Model file for the job. Use its own axes, mm. A direction names the side the tool comes from. Round coordinates to 2 decimals unless told otherwise and drop trailing zeros. Order: outer loops, then holes, each group sorted by start corner. A loop starts at its lowest first (then second) coordinate and runs counter-clockwise, first axis right, second up. Notation, with made-up numbers: (57, 10.25) - (69, 10.25) arc R19 ccw to (69, 23.25) - close; hole circle Ø10 at (47.25, 29). An arc over 180 degrees is marked (long way). Answer as CSV lines item,"result". Start each with the question number.
1. 3-axis set-ups, long thin cutter, end or side, ignore diameter. For faces 1 (the face through (-16.026, -11.579, 11.352)), 2 (the face through (-12.5, 0, 27)), 3 (the face through (12.5, 0, 27)): which of +Z, -Z, +X, -X, +Y, -Y reach the whole face in a straight line?
2. Pull direction Y, two halves, no side cores. Call faces 4 (the face through (0, 6.3, 27)), 5 (the face through (18.974, -11.579, 11.352)), 6 (the face through (-8.73, -11.89, 27.48)): released by +Y, released by -Y, zero draft, split by the parting line, or undercut.
3. Band-saw the part on C-C on y = -8.75. List the corners of the cut face in (x, z).
4. Band-saw the part on D-D on y = -5.2. List the corners of the cut face in (x, z).
5. Wall check: line 1 along Z through (x, y) = (-17.5, -10.5); line 2 along X through (y, z) = (-8.75, 37); line 3 along Y through (x, z) = (0, 30). Give the ranges that are in metal, low to high. Write a range as [from, to].
6. Band-saw the part on A-A on z = 10. List the corners of the cut face in (x, y).
7. Pin check, flat tips, straight feed: pin 1 Ø2 at (y, z) = (-3.5, 46) entering from +X; pin 2 Ø2.5 at (x, z) = (-17.5, 10) entering from +Y (3 decimals); pin 3 Ø6.5 at (y, z) = (-2.5, 19.5) entering from -X; pin 4 Ø3 at (x, z) = (15, 29.5) entering from +Y. Stop position of each tip, or through.
```python
from build123d import *

# Parameters (mm, degrees)
SKETCH1_W           = 25
SKETCH1_H           = 23
SKETCH1_R           = 11
SKETCH1_W_2         = 10
SKETCH1_H_2         = 10.1
BOSS_EXTRUDE1_DEPTH = 55.75
SKETCH2_R           = 2
CUT_EXTRUDE1_DEPTH  = 62.487580047


with BuildPart() as part:
    # Sketch1 → Boss-Extrude1 (new body)
    # profile 1 of 3: a face of its own
    with BuildSketch(Plane.XY):
        with Locations((0, -5.2)):
            Rectangle(SKETCH1_W, SKETCH1_H)
        with Locations((0, -5.2)):
            Circle(SKETCH1_R, mode=Mode.SUBTRACT)
    # profile 2 of 3: a face of its own
    with BuildSketch(Plane.XY):
        with Locations((-17.5, -11.65)):
            Rectangle(SKETCH1_W_2, SKETCH1_H_2)
    # profile 3 of 3: a face of its own
    with BuildSketch(Plane.XY):
        with Locations((17.5, -11.65)):
            Rectangle(SKETCH1_W_2, SKETCH1_H_2)
    extrude(amount=BOSS_EXTRUDE1_DEPTH)

    # Sketch2 → Cut-Extrude1 (cut, through all)
    with BuildSketch(Plane(origin=(0, -6.6, 0), x_dir=(1, 0, 0), z_dir=(0, 1, 0))):
        with Locations(Location((-17.5, -10, 0), (0, 0, 180))):
            Circle(SKETCH2_R)
        with Locations(Location((17.5, -10, 0), (0, 0, 180))):
            Circle(SKETCH2_R)
        with Locations(Location((-17.5, -37.75, 0), (0, 0, 180))):
            Circle(SKETCH2_R)
        with Locations(Location((17.5, -37.75, 0), (0, 0, 180))):
            Circle(SKETCH2_R)
    extrude(amount=-CUT_EXTRUDE1_DEPTH, mode=Mode.SUBTRACT)


solid = part.part
```
Reply:
1,face 1,"+Y, -Y"
1,face 2,"+Z, -Z, -X, +Y"
1,face 3,"+Z, -Z, +X, +Y"
2,face 4,"released by +Y"
2,face 5,"zero draft"
2,face 6,"undercut"
3,outline,"(-22.5, 0) - (-10.41, 0) - (-10.41, 55.75) - (-22.5, 55.75) - close; (10.41, 0) - (22.5, 0) - (22.5, 55.75) - (10.41, 55.75) - close; hole circle Ø4 at (-17.5, 10); hole circle Ø4 at (-17.5, 37.75); hole circle Ø4 at (17.5, 10); hole circle Ø4 at (17.5, 37.75)"
4,outline,"(-12.5, 0) - (-11, 0) - (-11, 55.75) - (-12.5, 55.75) - close; (11, 0) - (12.5, 0) - (12.5, 55.75) - (11, 55.75) - close"
5,line 1,"z = [0, 8], [12, 35.75], [39.75, 55.75]"
5,line 2,"x = [-22.5, -19.35], [-15.65, -10.41], [10.41, 15.65], [19.35, 22.5]"
5,line 3,"y = [-16.7, -16.2], [5.8, 6.3]"
6,outline,"(-22.5, -16.7) - (-19.5, -16.7) - (-19.5, -6.6) - (-22.5, -6.6) - close; (-15.5, -16.7) - (15.5, -16.7) - (15.5, -6.6) - (12.5, -6.6) - (12.5, 6.3) - (-12.5, 6.3) - (-12.5, -6.6) - (-15.5, -6.6) - close; (19.5, -16.7) - (22.5, -16.7) - (22.5, -6.6) - (19.5, -6.6) - close; hole circle Ø22 at (0, -5.2)"
7,pin 1,"stops at x = 12.5"
7,pin 2,"passes through"
7,pin 3,"stops at x = -12.5"
7,pin 4,"stops at y = -6.6"
